```python
from build123d import *

# Parameters (mm, degrees)
F0_R     = 6
F1_DEPTH = 2
F2_SIZE2 = 2.5980762114
F2_SIZE  = 1.5
F4_R     = 2.9
F4_R_2   = 1.4
F5_DEPTH = 4.5
F6_R     = 1.2


# Not quite as in the source:
# - a fillet or chamfer that OpenCascade refuses, or shapes differently, is made with other operations: its cross-section is extruded or revolved along the edge and cut away or added


with BuildPart() as f1:
    # F0 (on Top) → F1 (new body)
    with BuildSketch(Plane.XY):
        Circle(F0_R)
    extrude(amount=F1_DEPTH)

    # F2
    f2_edges = [f1.edges().sort_by_distance(p)[0] for p in [
        (-6, 0, 0),
    ]]
    f2_side = f1.faces().sort_by_distance((-6, 0, 1))[0]
    chamfer(f2_edges, length=F2_SIZE, length2=F2_SIZE2, reference=f2_side)

    # F3: fillet of radius 1 on 2 edges, made by hand

    # F3_s1 → F3_t2 (revolve, cut)
    with BuildSketch(Plane.XZ):
        with BuildLine():
            ThreePointArc((3.6339745962, 0.1339745962), (3.3927936413, 0.0340741737), (3.1339745962, 0))
            Line((3.1339745962, 0), (3.4019237886, 0))
            Line((3.4019237886, 0), (3.6339745962, 0.1339745962))
        make_face()
    revolve(axis=Axis((0, 0, 0), (0, 0, 1)), mode=Mode.SUBTRACT)

    # F3_s3 → F3_t4 (revolve, cut)
    with BuildSketch(Plane.XZ):
        with BuildLine():
            ThreePointArc((6, 2), (5.8486778537, 1.5452494356), (5.5031382462, 1.2131367327))
            Line((5.5031382462, 1.2131367327), (6, 1.5))
            Line((6, 1.5), (6, 2))
        make_face()
    revolve(axis=Axis((0, 0, 1.5), (0, 0, 1)), mode=Mode.SUBTRACT)

    # F4 (on face) → F5 (join)
    with BuildSketch(Plane.XY.offset(2)):
        Circle(F4_R)
        Circle(F4_R_2, mode=Mode.SUBTRACT)
    extrude(amount=F5_DEPTH)

    # F6
    f6_edges = [f1.edges().sort_by_distance(p)[0] for p in [
        (-1.4, 0, 2),
    ]]
    fillet(f6_edges, radius=F6_R)


solid = f1.part
```
Model file for the job. Use its own axes, mm. Coordinates: 2 decimals unless noted, no trailing zeros. Write each loop counter-clockwise with the first axis right and the second up, starting at its lowest first coordinate (ties: lowest second). Pieces come first, ordered by that corner, then holes. Notation, with made-up numbers: (-38.5, 65.5) - (8.5, 65.5) arc R34 ccw to (8.5, 104.5) - close; hole circle Ø9 at (78, -34). An arc over 180 degrees is marked (long way). Use a Markdown table: item, result. Add a question column.
Item 1: Two-plate mould, pull along X, no slides. Class faces 1 (the face through (-2.9, 0.1, 4.2)), 2 (the face through (-1.4, 0.06, 4.83)), 3 (the face through (3, 1, 2)): pulls with the +X half, pulls with the -X half, needs draft (parallel to the pull), parting line crosses it, or undercut.
Item 2: Drill centre lines: line 1 along Y through (x, z) = (0, 5); line 2 along Y through (x, z) = (-1, 2.5); line 3 along Z through (x, y) = (-3.75, -3.25). Where is each one in solid material? Low to high.
Item 3: Band-saw the part on A-A, the plane z = 5.5. Write the cut outline in (x, y).
Item 4: Drop flat-ended pins along their axis: pin 1 (2 mm diameter, centred on x = -3, z = 4.5, fed in from +Y); pin 2 (2 mm diameter, centred on y = -1.5, z = 5, fed in from +X); pin 3 (1 mm diameter, centred on x = 2.5, z = 2, fed in from -Y). Give the stop position or say it passes through.
Item 5: Band-saw the part on B-B, the plane z = 0.5. Write the cut outline in (x, y), and give its area (3 significant figures).
A:
| question | item | result |
|---|---|---|
| 1 | face 1 | parting line crosses it |
| 1 | face 2 | undercut |
| 1 | face 3 | needs draft |
| 2 | line 1 | y = -2.9 to -1.4, 1.4 to 2.9 |
| 2 | line 2 | y = -2.72 to -0.62, 0.62 to 2.72 |
| 2 | line 3 | z = 0.9 to 2 |
| 3 | outline | circle Ø5.8 at (0, 0); hole circle Ø2.8 at (0, 0) |
| 4 | pin 1 | stops at y = 2.1 |
| 4 | pin 2 | stops at x = 2.86 |
| 4 | pin 3 | stops at y = -5.66 |
| 5 | outline | circle Ø8.54 at (0, 0) |
| 5 | area | 57.2 mm² |
